Model file for the job. Use its own axes, mm. Give positions to 0.01 mm unless a question says otherwise; leave off trailing zeros. Order: outer loops, then holes, each group sorted by start corner. A loop starts at its lowest first (then second) coordinate and runs counter-clockwise, first axis right, second up. Notation, with made-up numbers: M 55,49.5 L 84,49.5 A21 cw 84,55.5 Z; hole C -14.75,40 d3. An arc over 180 degrees is marked long. Return JSON: item names as keys, results as strings. Group by question number.
1. Pin check, flat tips, straight feed: pin 1 (4 mm diameter, centred on y = 17, z = -137.5, fed in from -X); pin 2 (9 mm diameter, centred on y = 15.5, z = -113, fed in from +X). Stop position of each tip, or through.
2. Wall check: probe 1 along Z at (x, y) = (-65, 15.25) (3 decimals); probe 2 along X at (y, z) = (20.25, -46); probe 3 along Y at (x, z) = (60, -233.5) (3 decimals). Give the ranges that are in metal, low to high. Write a range as [from, to].
3. Slice it at A-A on z = -109.5. List the corners of the cut face in (x, y) (1 decimal), then the cut area to 3 significant figures.
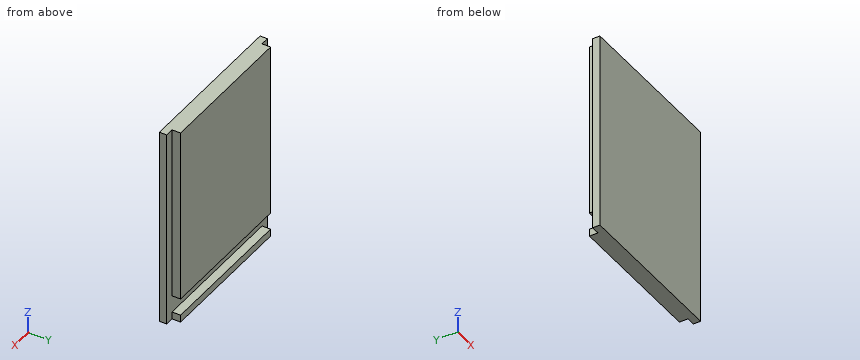
from build123d import *

# Parameters (mm, degrees)
F0_W     = 209.55
F0_H     = 20.6375
F1_DEPTH = 260.35
F2_W     = 209.55
F2_H     = 22.225
F3_DEPTH = 11.1125
F4_W     = 11.1125
F4_H     = 11.1125
F5_DEPTH = 260.351


# Not quite as in the source:
# - a length typed as a fraction of an inch, garbled in the dataset ("3 / 203.2 mm" for 3/8 in), is restored


with BuildPart() as f1:
    # F0 (on Top) → F1 (new body)
    with BuildSketch(Plane.XY):
        with Locations((0, 10.31875)):
            Rectangle(F0_W, F0_H)
    extrude(amount=-F1_DEPTH)

    # F2 (on face) → F3 (cut)
    with BuildSketch(Plane(origin=(0, 20.6375, 0), x_dir=(-1, 0, 0), z_dir=(0, 1, 0))):
        with Locations((0, -239.7125)):
            Rectangle(F2_W, F2_H)
    extrude(amount=-F3_DEPTH, mode=Mode.SUBTRACT)

    # F4 (on face) → F5 (cut, through all)
    with BuildSketch(Plane(origin=(0, 0, -260.35), x_dir=(1, 0, 0), z_dir=(0, 0, -1))):
        with Locations((-99.21875, -15.08125)):
            Rectangle(F4_W, F4_H)
        with Locations((99.21875, -15.08125)):
            Rectangle(F4_W, F4_H)
    extrude(amount=-F5_DEPTH, mode=Mode.SUBTRACT)


solid = f1.part
Result:
{
 "1": {"pin 1": "stops at x = -93.66", "pin 2": "stops at x = 93.66"},
 "2": {"probe 1": "z = [-260.35, -250.825], [-228.6, 0]", "probe 2": "x = [-93.66, 93.66]", "probe 3": "y = [0, 9.525]"},
 "3": {"outline": "M -104.8,0 L 104.8,0 L 104.8,9.5 L 93.7,9.5 L 93.7,20.6 L -93.7,20.6 L -93.7,9.5 L -104.8,9.5 Z", "area": "4,080 mm2"}
}
